```python
from build123d import *

# Parameters (mm, degrees)
F0_R      = 67
F1_DEPTH  = 2.5
F3_R      = 64.375
F3_R_2    = 62.625
F4_DEPTH  = 3
F5_R      = 62.625
F5_R_2    = 58.875
F6_DEPTH  = 2
F7_R      = 4.25
F8_DEPTH  = 5.001
F9_R      = 5.75
F10_DEPTH = 5.001
F11_R     = 5.75
F12_DEPTH = 5.001
F14_R     = 2.1
F15_DEPTH = 5.001
F16_R     = 5.25
F18_DEPTH = 0.5
F19_R     = 6.75
F20_DEPTH = 0.5
F11_R_2   = 6.75
F21_DEPTH = 0.5
F22_DEPTH = 3


with BuildPart() as f1:
    # F0 (on Top) → F1 (new body, symmetric)
    with BuildSketch(Plane.XY):
        Circle(F0_R)
    extrude(amount=F1_DEPTH, both=True)

    # F3 (on face) → F4 (join)
    with BuildSketch(Plane.XY.offset(2.5)):
        Circle(F3_R)
        Circle(F3_R_2, mode=Mode.SUBTRACT)
    extrude(amount=F4_DEPTH)

    # F5 (on face) → F6 (cut)
    with BuildSketch(Plane.XY.offset(2.5)):
        Circle(F5_R)
        Circle(F5_R_2, mode=Mode.SUBTRACT)
    extrude(amount=-F6_DEPTH, mode=Mode.SUBTRACT)

    # F7 (on face) → F8 (cut, through all)
    with BuildSketch(Plane.XY.offset(2.5)):
        Circle(F7_R)
    extrude(amount=-F8_DEPTH, mode=Mode.SUBTRACT)

    # F9 (on face) → F10 (cut, through all)
    with BuildSketch(Plane.XY.offset(2.5)):
        with Locations((0, 18.75)):
            Circle(F9_R)
    extrude(amount=-F10_DEPTH, mode=Mode.SUBTRACT)

    # F11 (on face) → F12 (cut, through all)
    with BuildSketch(Plane.XY.offset(2.5)):
        with Locations((0, 46.25)):
            Circle(F11_R)
    extrude(amount=-F12_DEPTH, mode=Mode.SUBTRACT)

    # F14 (on face) → F15 (cut, through all)
    with BuildSketch(Plane.XY.offset(2.5)):
        with Locations((-17.709117, -8)):
            Circle(F14_R)
        with Locations((17.709117, -8)):
            Circle(F14_R)
    extrude(amount=-F15_DEPTH, mode=Mode.SUBTRACT)

    # F16 (on face) → F18 (cut)
    with BuildSketch(Plane.XY.offset(2.5)):
        Circle(F16_R)
    extrude(amount=-F18_DEPTH, mode=Mode.SUBTRACT)

    # F19 (on face) → F20 (cut)
    with BuildSketch(Plane.XY.offset(2.5)):
        with Locations((0, 18.75)):
            Circle(F19_R)
    extrude(amount=-F20_DEPTH, mode=Mode.SUBTRACT)

    # F11 (on face) → F21 (cut)
    with BuildSketch(Plane.XY.offset(2.5)):
        with Locations((0, 46.25)):
            Circle(F11_R_2)
        with Locations((0, 46.25)):
            Circle(F11_R, mode=Mode.SUBTRACT)
    extrude(amount=-F21_DEPTH, mode=Mode.SUBTRACT)

    # F17 (on face) → F22 (cut)
    with BuildSketch(Plane.XY.offset(2.5)):
        Polygon((-13.75, -10.165064), (-13.75, -5.834936), (-17.5, -3.669873), (-21.25, -5.834936), (-21.25, -10.165064), (-17.5, -12.330127), align=None)
        Polygon((21.25, -10.165064), (21.25, -5.834936), (17.5, -3.669873), (13.75, -5.834936), (13.75, -10.165064), (17.5, -12.330127), align=None)
    extrude(amount=-F22_DEPTH, mode=Mode.SUBTRACT)


solid = f1.part
```
Design review of the part built by this model. Coordinates are the model's own, in mm. A direction names the side the tool comes from. Round coordinates to 2 decimals unless told otherwise and drop trailing zeros. Write each loop counter-clockwise with the first axis right and the second up, starting at its lowest first coordinate (ties: lowest second). Pieces come first, ordered by that corner, then holes. Notation, with made-up numbers: (63, -19) -> (110, -19) arc R30 ccw to (110, 8) -> close; hole circle Ø2 at (4, 72.5). An arc over 180 degrees is marked (long way). Write item = value, one per line. Start each with the question number.
1) Take a section at B-B, the plane x = 0. Count the separate pieces of the cut face and the enclosed holes in it, plus the area to 3 significant figures.
2) Take a section at A-A, the plane y = 46.25. State the section outline as (x, z) points.
3) Tool access review of faces 4 (the face through (19.712, -7.369, -1.486)), 5 (the face through (46, -37, 0.5)): name each direction out of +Z, -Z, +X, -X, +Y, -Y from which nothing blocks a thin tool from reaching the whole face with its end or side.
4) Clearance check with flat-ended pins moving along their axes: pin 1 (1.5 mm diameter, centred on y = -9, z = 1, fed in from -X); pin 2 (1.5 mm diameter, centred on x = -24.5, y = 44.5, fed in from +Z); pin 3 (1.5 mm diameter, centred on x = 37.5, z = 3.5, fed in from -Y). State where each tip first meets the part, or that it passes through.
5) Mouldability with a two-part tool opening along X and no side actions: class faces 1 (the face through (-14.524, -65.407, 0.035)), 2 (the face through (13.75, -8, 1)), 3 (the face through (14, -62, 5.5)) as +X half, -X half, draft (parallel to the pull), parting line (faces both ways), or undercut.
6) Wall thickness on probe 1 along X at (y, z) = (-0.5, 1.5); probe 2 along Y at (x, z) = (0, 2.3) (3 decimals); probe 3 along Y at (x, z) = (0, 4.3) (3 decimals): over which ranges is each line inside the solid? List them lowest first. Write a range as from..to.
7) Take a section at D-D, the plane y = -57. State the section outline as (x, z) points, plus the area to 3 significant figures.
Results list:
q1.separate_pieces = 4
q1.enclosed_holes = 0
q1.area = 505 mm²
q2.outline = (-48.48, -2.5) -> (-5.75, -2.5) -> (-5.75, 2) -> (-6.75, 2) -> (-6.75, 2.5) -> (-36.43, 2.5) -> (-36.43, 0.5) -> (-42.22, 0.5) -> (-42.22, 5.5) -> (-44.78, 5.5) -> (-44.78, 2.5) -> (-48.48, 2.5) -> close; (5.75, -2.5) -> (48.48, -2.5) -> (48.48, 2.5) -> (44.78, 2.5) -> (44.78, 5.5) -> (42.22, 5.5) -> (42.22, 0.5) -> (36.43, 0.5) -> (36.43, 2.5) -> (6.75, 2.5) -> (6.75, 2) -> (5.75, 2) -> close
q3.face_4 = +Z, -Z
q3.face_5 = +Z
q4.pin_1 = -66.49
q4.pin_2 = 2.5
q4.pin_3 = -52.85
q5.face_1 = parting line
q5.face_2 = undercut
q5.face_3 = draft
q6.probe_1 = -67..-62.62, -58.87..-4.22, 4.22..58.87, 62.62..67
q6.probe_2 = -67..-62.625, -58.875..-5.25, 5.25..12, 25.5..39.5, 53..58.875, 62.625..67
q6.probe_3 = -64.375..-62.625, 62.625..64.375
q7.outline = (-35.21, -2.5) -> (35.21, -2.5) -> (35.21, 2.5) -> (29.92, 2.5) -> (29.92, 5.5) -> (25.94, 5.5) -> (25.94, 0.5) -> (14.74, 0.5) -> (14.74, 2.5) -> (-14.74, 2.5) -> (-14.74, 0.5) -> (-25.94, 0.5) -> (-25.94, 5.5) -> (-29.92, 5.5) -> (-29.92, 2.5) -> (-35.21, 2.5) -> close
q7.area = 331 mm²
